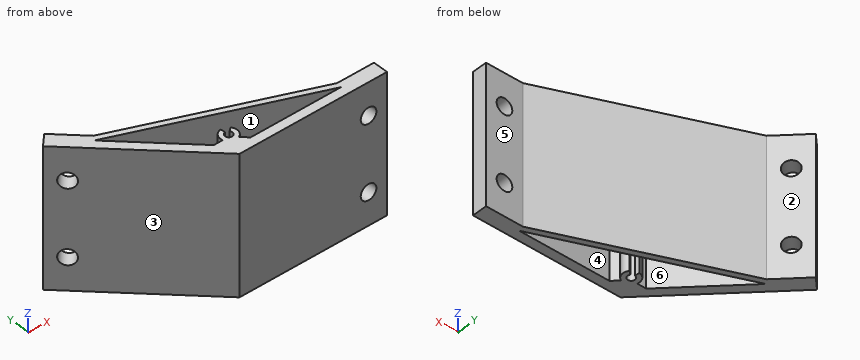
```python
from build123d import *

# Parameters (mm, degrees)
EXTRUDE_1_DEPTH         = 37.5
HOLE_WIZARD_8_5_8_5_1_D = 8.5
HOLE_WIZARD_8_5_8_5_2_D = 8.5


with BuildPart() as part:
    # 草图1 → 凸台-拉伸1 (new, symmetric)
    with BuildSketch(Plane.XY):
        Polygon((6936.119122288, -1232.086390659), (6992.687664783, -1288.654933154), (7072.687664783, -1288.654933154), (7072.687664783, -1280.654933154), (7052.687664783, -1280.654933154), (6955.918112162, -1240.571672033), (6941.775976538, -1226.429536409), align=None)
        with BuildLine():
            Line((7009.090927681, -1283.654933154), (7003.090927681, -1283.654933154))
            Line((7003.090927681, -1283.654933154), (6999.760549745, -1280.324555218))
            ThreePointArc((6999.760549745, -1280.324555218), (7002.213755914, -1277.239517812), (7001.296666197, -1273.406161221))
            Line((7001.296666197, -1273.406161221), (6999.365595427, -1274.993916141))
            ThreePointArc((6999.365595427, -1274.993916141), (6997.055371947, -1278.111879141), (6997.626530039, -1274.273571671))
            Line((6997.626530039, -1274.273571671), (6997.383769074, -1271.785386165))
            ThreePointArc((6997.383769074, -1271.785386165), (6994.101203016, -1273.731324494), (6993.49338103, -1277.49861375))
            Line((6993.49338103, -1277.49861375), (6988.602413191, -1277.49861375))
            Line((6988.602413191, -1277.49861375), (6954.21874867, -1243.114949228))
            Line((6954.21874867, -1243.114949228), (7052.090927681, -1283.654933154))
            Line((7052.090927681, -1283.654933154), (7029.403393536, -1283.654933154))
            Line((7029.403393536, -1283.654933154), (7009.090927681, -1283.654933154))
        make_face(mode=Mode.SUBTRACT)
    extrude(amount=EXTRUDE_1_DEPTH, both=True)

    # Ø8.5 (8.5) 直径孔1 (through all)
    with Locations(Plane(origin=(2852.016365815, 2852.016365815, 0), x_dir=(0.7071067811865628, -0.7071067811865324, 0), z_dir=(-0.7071067811865324, -0.7071067811865628, 0))):
        with Locations((5785.79350833, -20), (5785.79350833, 20)):
            Hole(HOLE_WIZARD_8_5_8_5_1_D / 2)

    # Ø8.5 (8.5) 直径孔2 (through all)
    with Locations(Plane.XZ.offset(1288.654933154)):
        with Locations((7062.687664783, -20), (7062.687664783, 20)):
            Hole(HOLE_WIZARD_8_5_8_5_2_D / 2)


solid = part.part
```
Verification items for the finished model (mm, model axes). Face numbers are marked on the shaded views. A direction names the side the tool comes from. Coordinates: 2 decimals unless noted, no trailing zeros. Write each loop counter-clockwise with the first axis right and the second up, starting at its lowest first coordinate (ties: lowest second). Pieces come first, ordered by that corner, then holes. Notation, with made-up numbers: M 4.5,-25.75 L 62.5,-25.75 A19 cw 62.5,-21.75 Z; hole C 29.5,-34.5 d11. An arc over 180 degrees is marked long. One line per item, written item: value.
Item 1: Section check C-C, the plane z = 20. Record the boundary of the cut face in (x, y).
Check sheet entries:
outline: M 6936.12,-1232.09 L 6940.18,-1236.15 L 6945.84,-1230.5 L 6941.78,-1226.43 Z; M 6946.2,-1242.16 L 6992.69,-1288.65 L 7058.44,-1288.65 L 7058.44,-1280.65 L 7052.69,-1280.65 L 6955.92,-1240.57 L 6951.85,-1236.51 Z; M 7066.94,-1288.65 L 7072.69,-1288.65 L 7072.69,-1280.65 L 7066.94,-1280.65 Z; hole M 6954.22,-1243.11 L 6988.6,-1277.5 L 6993.49,-1277.5 A4.5 cw 6997.38,-1271.79 L 6997.63,-1274.27 A2 ccw long 6999.37,-1274.99 L 7001.3,-1273.41 A4.5 cw 6999.76,-1280.32 L 7003.09,-1283.65 L 7052.09,-1283.65 Z
Item 2: Section check D-D, the plane y = -1270. Record the boundary of the cut face in (x, z) (3 decimals).
Check sheet entries:
outline: M 6974.033,-37.5 L 6981.104,-37.5 L 6981.104,37.5 L 6974.033,37.5 Z; M 7019.125,-37.5 L 7026.964,-37.5 L 7026.964,37.5 L 7019.125,37.5 Z
Item 3: Section check B-B, the plane x = 7011. Record the boundary of the cut face in (y, z).
Check sheet entries:
outline: M -1288.65,-37.5 L -1283.65,-37.5 L -1283.65,37.5 L -1288.65,37.5 Z; M -1266.63,-37.5 L -1263.39,-37.5 L -1263.39,37.5 L -1266.63,37.5 Z
Item 4: Section check A-A, the plane z = 11. Record the boundary of the cut face in (x, y), plus the area to 3 significant figures.
Check sheet entries:
outline: M 6936.12,-1232.09 L 6992.69,-1288.65 L 7072.69,-1288.65 L 7072.69,-1280.65 L 7052.69,-1280.65 L 6955.92,-1240.57 L 6941.78,-1226.43 Z; hole M 6954.22,-1243.11 L 6988.6,-1277.5 L 6993.49,-1277.5 A4.5 cw 6997.38,-1271.79 L 6997.63,-1274.27 A2 ccw long 6999.37,-1274.99 L 7001.3,-1273.41 A4.5 cw 6999.76,-1280.32 L 7003.09,-1283.65 L 7052.09,-1283.65 Z
area: 1,310 mm^2
Item 5: Mould release check, pull along X, two halves, no side actions. Record for the marked faces 3, 4, 5 and 6: pulls with the +X half, pulls with the -X half, needs draft (parallel to the pull), parting line crosses it, or undercut.
Check sheet entries:
face 3: pulls with the -X half
face 4: undercut
face 5: needs draft
face 6: undercut
Item 6: Scan lines: line 1 along X through (y, z) = (-1277, 21.5); line 2 along X through (y, z) = (-1278, 28.5); line 3 along Y through (x, z) = (7041, 9). Record each from-to range of solid material in increasing order.
Check sheet entries:
line 1: x = 6981.03 to 6988.1, 6993.38 to 6995.96, 6999.68 to 7002.26, 7036.02 to 7043.86
line 2: x = 6982.03 to 6996.83, 6998.81 to 7001.97, 7038.44 to 7046.28
line 3: y = -1288.65 to -1283.65, -1279.06 to -1275.81
Item 7: Access from +Z, -Z, +X, -X, +Y, -Y to the whole of each face (thin tool, end or side, straight path). Record for the marked faces 1 and 2.
Check sheet entries:
face 1: +Z, -Z
face 2: +Z, -Z, +X, +Y
Item 8: Gauge pin test, flat ends, axial feed: pin 1 Ø6 at (x, y) = (7038.5, -1268.5) entering from +Z; pin 2 Ø10 at (y, z) = (-1269.5, 12) entering from +X; pin 3 Ø5 at (x, z) = (6950.5, 16.5) entering from -Y; pin 4 Ø4 at (y, z) = (-1241.5, 6.5) entering from -X. Record the tip position at first contact, or that the pin passes through.
Check sheet entries:
pin 1: passes through
pin 2: stops at x = 7037.83
pin 3: stops at y = -1248.97
pin 4: stops at x = 6943.53
